Answer from the drawing. Dimensions are ordinates in mm from the lowest x, y and z of the part. Give positions to 0.01 mm unless a question says otherwise; leave off trailing zeros. Loops run counter-clockwise (first coordinate to the right, second up) from the corner with the lowest first, then second, coordinate; pieces in that order, holes last. Notation, with made-up numbers: (86.25, 42.5) - (143.25, 42.5) arc R29 cw to (143.25, 78.5) - close; hole circle Ø3 at (88, 22). An arc over 180 degrees is marked (long way). Write each question's results on one line, items separated by ' | '. Start each with the question number.
Q1. The part is cut by section C-C, the plane z = 3.85. Write down the section's boundary in (x, y).
Q2. Given pin 1 (5 mm diameter, centred on x = 57.5, y = 37.5, fed in from -Z); pin 2 (1.5 mm diameter, centred on x = 21.5, z = 1, fed in from -Y); pin 3 (2 mm diameter, centred on y = 20, z = 2.5, fed in from +X), each flat-ended and moving along its own axis, determine where each tip first touches the part or whether it passes through.
Q3. Find the intervals of material crossed by line 1 (Y direction, x = 33, z = 2.55); line 2 (Y direction, x = 47.5, z = 4.35); line 3 (X direction, y = 57.5, z = 1.8), in increasing order. Write a range as from..to.
Q4. The part is cut by section A-A, the plane y = 33. Write down the section's boundary in (x, z).
Q5. Determine the mould class of the marked faces 1, 2 and 3 for opening direction Y: +Y half, -Y half, draft (parallel to the pull), parting line (faces both ways), or undercut.
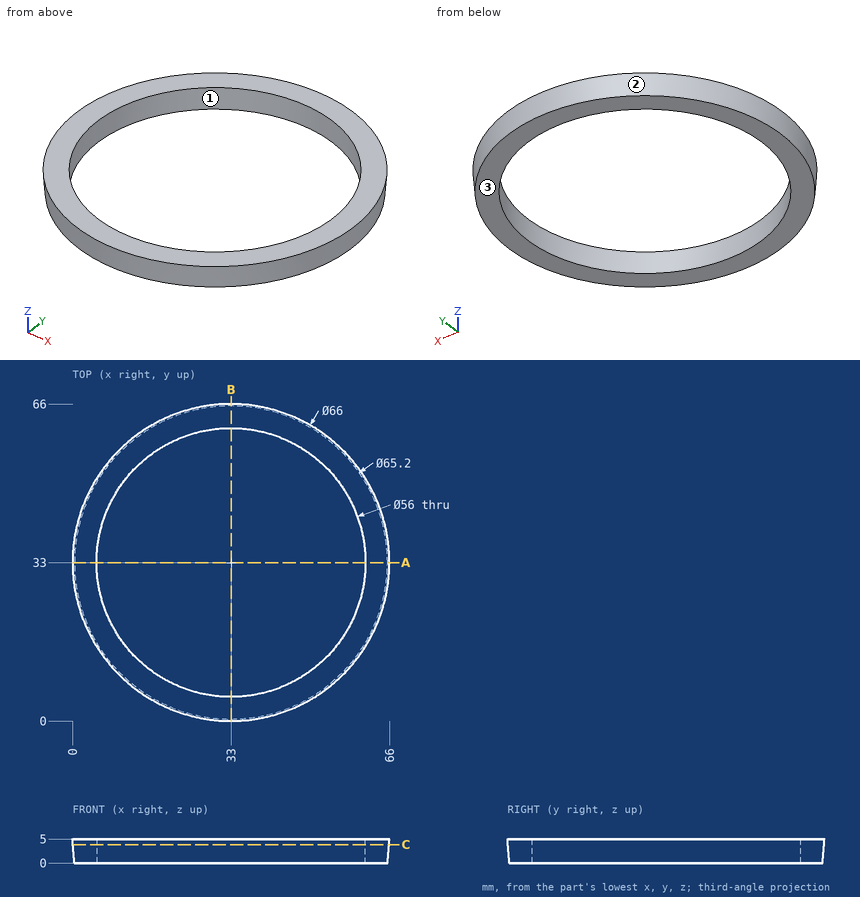
Check sheet entries:
1) outline: circle Ø65.82 at (33, 33); hole circle Ø56 at (33, 33)
2) pin 1: passes through | pin 2: stops at y = 2.13 | pin 3: stops at x = 63.54
3) line 1: y = 0.2..5, 61..65.8 | line 2: y = 3.41..9.05, 56.95..62.59 | line 3: x = 11.28..19.44, 46.56..54.72
4) outline: (0, 5) - (0.4, 0) - (5, 0) - (5, 5) - close; (61, 0) - (65.6, 0) - (66, 5) - (61, 5) - close
5) face 1: undercut | face 2: parting line | face 3: draft
